Solid Edge part; units mm, degrees
sketch "Sketch1" plane through (0, 0, 0) normal (0, -1, 0) x (1, 0, 0)
  line L0 (-30, 0) -> (30, 0)
  line L1 (30, 0) -> (30, 30)
  line L2 (30, 30) -> (15, 40)
  arc A0 (-15, 40) -> (15, 40) centre (0, 40) cw
  line L3 (-30, 30) -> (-15, 40)
  line L4 (-30, 0) -> (-30, 30)
  dimension "D1" = 30
  dimension "D2" = 30
extrude "Protrusion1" add sketch "Sketch1" along normal mid plane 12
hole "Hole_1" at (0, -6, 40) direction (0, 1, 0) diameter 5 end up to next
hole "Hole_2" at (-20, 0, 40) direction (0, 0, -1) diameter 4.8 end up to next counterbore diameter 9 counterbore depth 22
hole "Hole1" at (20, 0, 40) direction (0, 0, -1) diameter 4.8 end up to next counterbore diameter 9 counterbore depth 22
sketch "Sketch2" plane through (0, 6, 20) normal (0, 1, 0) x (-1, 0, 0)
  line L0 (-30, -10) -> (30, -10)
extrude "ExtrudedCutout_1" cut sketch "Sketch2" against normal blind 3 material side at (0, 6, 10.05)
sketch "Sketch3" plane through (0, 0, 0) normal (0, 0, -1) x (1, 0, 0)
  arc A0 (-30, 6) -> (30, 6) centre (0, -34) cw
  line L0 (-30, 6) -> (30, 6)
extrude "ExtrudedProtrusion_2" add sketch "Sketch3" against normal blind 25
chamfer "Chamfer_1" distance 8 angle 45 1 edges at (0, -16, 25)
properties material "Polyethylene, low density"
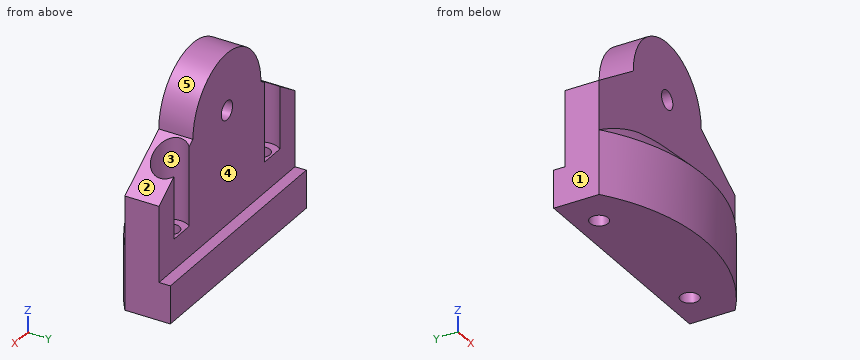
Read the model definition and answer for the solid it produces. Units are mm, in the model's axes. Face numbers are marked on the shaded views. A direction names the side the tool comes from. Coordinates: 2 decimals unless noted, no trailing zeros. Write each loop counter-clockwise with the first axis right and the second up, starting at its lowest first coordinate (ties: lowest second). Pieces come first, ordered by that corner, then holes. Notation, with made-up numbers: (7.25, 84) - (61.25, 84) arc R33 cw to (61.25, 117) - close; hole circle Ø7 at (-35.75, -23). An arc over 180 degrees is marked (long way). Answer as a JSON object with one key per item and string values. Group by question number.
1. Each of these flat-tipped pins is pushed along its axis until it touches: P1, Ø4.5, axis at x = 0, z = 40, coming from the -Y side; P2, Ø8, axis at x = -16, z = 17.5, coming from the +Y side; P3, Ø1.5, axis at x = 14, z = 41, coming from the -Y side; P4, Ø4, axis at x = -7, y = 1, coming from the +Z side. Where does it stop, or does it pass through?
2. A cutting plane is placed at D-D (z = 26). Determine the outline of the cut face in (x, y), plus the area to 3 significant figures.
3. A cutting plane is placed at B-B (y = 0). Determine the outline of the cut face in (x, z).
4. A cutting plane is placed at A-A (x = 0). Determine the outline of the cut face in (y, z), plus the area to 3 significant figures.
5. Consider L1, parallel to X at y = 0, z = 5.5; L2, parallel to X at y = 0, z = 23.75; L3, parallel to Y at x = -20, z = 12.25. Determine where each line is inside the solid, lowest interval first. Write a range as [from, to].
6. A cutting plane is placed at C-C (z = 7.5). Determine the outline of the cut face in (x, y).
7. The mould has two halves that part along X. Classify the marked faces 1, 2 and 3: +X half, -X half, draft (parallel to the pull), parting line (faces both ways), or undercut.
8. Which of the six approach directions +Z, -Z, +X, -X, +Y, -Y give full straight-line access (tool end or side, diameter ignored) to the marked faces 4 and 5?
Worked out:
{
 "1": {"P1": "passes through", "P2": "stops at y = 3", "P3": "stops at y = -6", "P4": "stops at z = 54.14"},
 "2": {"outline": "(-30, -6) - (30, -6) - (30, 3) - (23.35, 3) arc R4.5 cw (long way) to (16.65, 3) - (-16.65, 3) arc R4.5 cw (long way) to (-23.35, 3) - (-30, 3) - close", "area": "427 mm²"},
 "3": {"outline": "(-30, 0) - (-22.4, 0) - (-22.4, 18) - (-24.5, 18) - (-24.5, 33.67) - (-30, 30) - close; (-17.6, 0) - (17.6, 0) - (17.6, 18) - (15.5, 18) - (15.5, 39.67) - (15, 40) arc R15 ccw to (-15, 40) - (-15.5, 39.67) - (-15.5, 18) - (-17.6, 18) - close; (22.4, 0) - (30, 0) - (30, 30) - (24.5, 33.67) - (24.5, 18) - (22.4, 18) - close; hole circle Ø5 at (0, 40)"},
 "4": {"outline": "(-16, 0) - (6, 0) - (6, 10) - (3, 10) - (3, 37.5) - (-6, 37.5) - (-6, 25) - (-8, 25) - (-16, 17) - close; (-6, 42.5) - (3, 42.5) - (3, 55) - (-6, 55) - close", "area": "698 mm²"},
 "5": {"L1": "x = [-30, -22.4], [-17.6, 17.6], [22.4, 30]", "L2": "x = [-30, -24.5], [-15.5, 15.5], [24.5, 30]", "L3": "y = [-11.83, -2.4], [2.4, 3]"},
 "6": {"outline": "(-30, -6) arc R50 ccw to (30, -6) - (30, 6) - (-30, 6) - close; hole circle Ø4.8 at (-20, 0); hole circle Ø4.8 at (20, 0)"},
 "7": {"face 1": "-X half", "face 2": "+X half", "face 3": "undercut"},
 "8": {"face 4": "+Z, +X, -X, +Y", "face 5": "+Z, +Y, -Y"}
}
